Design review of the part shown in the three views and the two pictorial views. Dimensions are in mm from the part's minimum x, y and z. A direction names the side the tool comes from. Give positions to 0.01 mm unless a question says otherwise; leave off trailing zeros. Write each loop counter-clockwise with the first axis right and the second up, starting at its lowest first coordinate (ties: lowest second). Pieces come first, ordered by that corner, then holes. Notation, with made-up numbers: (35, 85.25) -> (43, 85.25) arc R27 cw to (43, 114.25) -> close; hole circle Ø10 at (62, 21.5). An arc over 180 degrees is marked (long way). Return JSON: item names as keys, results as strings. Group by question number.
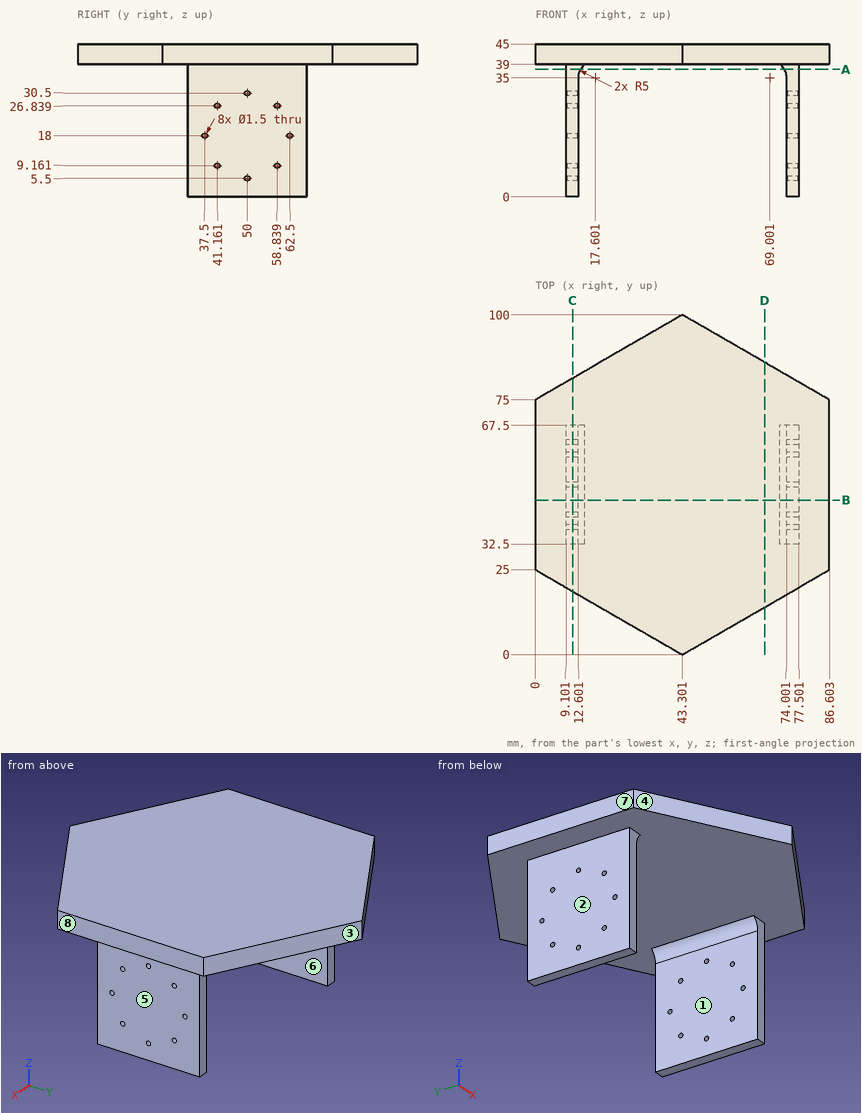
Q1. Take a section at C-C, the plane x = 11. Count the separate pieces of the cut face and the enclosed holes in it, plus the area to 3 significant figures.
Q2. Mouldability with a two-part tool opening along X and no side actions: class the marked faces 6, 7 and 8 as +X half, -X half, draft (parallel to the pull), parting line (faces both ways), or undercut.
Q3. Tool access review of the marked faces 1, 2, 3, 4 and 5: name each direction out of +Z, -Z, +X, -X, +Y, -Y from which nothing blocks a thin tool from reaching the whole face with its end or side.
Q4. Take a section at D-D, the plane x = 67.5. Give the boundary of the cut face in (y, z).
Q5. Take a section at A-A, the plane z = 37.5. Give the boundary of the cut face in (x, y).
Q6. For L1, parallel to Z at x = 75.7, y = 50; L2, parallel to Y at x = 75.65, z = 18; L3, parallel to Y at x = 10.6, z = 5.5, list the stretches that pass through material, from the lowest coordinate up. Write a range as from..to.
Q7. Take a section at B-B, the plane y = 45.5. Give the boundary of the cut face in (x, z).
Q8. Insertion check: pin 1 (1.7 mm diameter, centred on y = 50, z = 30.5, fed in from +X); pin 2 (4 mm diameter, centred on y = 69, z = 26, fed in from -X); pin 3 (2 mm diameter, centred on x = 55.5, y = 81.5, fed in from -Z). Each pin has a flat end and moves straight along its axis. Give the tip position at first contact, or say it passes through.
Final values:
{
 "1": {"separate pieces": "1", "enclosed holes": "8", "area": "1,730 mm²"},
 "2": {"face 6": "undercut", "face 7": "-X half", "face 8": "+X half"},
 "3": {"face 1": "-Z, +Y, -Y", "face 2": "-Z, -X, +Y, -Y", "face 3": "+Z, -Z, +X, +Y", "face 4": "+Z, -Z, -X, -Y", "face 5": "-Z, +X, +Y, -Y"},
 "4": {"outline": "(13.97, 39) -> (86.03, 39) -> (86.03, 45) -> (13.97, 45) -> close"},
 "5": {"outline": "(9.1, 32.5) -> (13.27, 32.5) -> (13.27, 67.5) -> (9.1, 67.5) -> close; (73.33, 32.5) -> (77.5, 32.5) -> (77.5, 67.5) -> (73.33, 67.5) -> close"},
 "6": {"L1": "z = 0..4.75, 6.25..29.75, 31.25..45", "L2": "y = 32.5..36.75, 38.25..61.75, 63.25..67.5", "L3": "y = 32.5..49.25, 50.75..67.5"},
 "7": {"outline": "(0, 39) -> (9.1, 39) -> (9.1, 0) -> (12.6, 0) -> (12.6, 35) arc R5 cw to (14.6, 39) -> (72, 39) arc R5 cw to (74, 35) -> (74, 0) -> (77.5, 0) -> (77.5, 39) -> (86.6, 39) -> (86.6, 45) -> (0, 45) -> close"},
 "8": {"pin 1": "stops at x = 77.5", "pin 2": "stops at x = 9.1", "pin 3": "stops at z = 39"}
}
